Read the model definition and answer for the solid it produces. Units are mm, in the model's axes. Face numbers are marked on the shaded views. A direction names the side the tool comes from. Coordinates: 2 decimals unless noted, no trailing zeros. Loops run counter-clockwise (first coordinate to the right, second up) from the corner with the lowest first, then second, coordinate; pieces in that order, holes last. Notation, with made-up numbers: (69.5, -15.5) - (91.5, -15.5) arc R30 ccw to (91.5, 10.5) - close; hole circle Ø3 at (39, 44.5). An arc over 180 degrees is marked (long way). Use one line per item in the form item = value. Start each with the question number.
1) A cutting plane is placed at C-C (z = 6). State how many separate pieces and enclosed holes the cut face has, and give its area (3 significant figures).
2) A cutting plane is placed at A-A (y = 10). Give the vertices of the cut face in (x, z) (1 decimal).
3) The mould has two halves that part along X. Classify the marked faces 1, 2 and 3: released by +X, released by -X, zero draft, split by the parting line, or undercut.
4) Which of the six approach directions +Z, -Z, +X, -X, +Y, -Y give full straight-line access (tool end or side, diameter ignored) to the marked faces 4, 5 and 6?
5) A cutting plane is placed at B-B (y = 21.75). Give the vertices of the cut face in (x, z).
6) Consider line 1 (X direction, y = 16.5, z = 3); line 2 (X direction, y = 6.5, z = 6); line 3 (Z direction, x = 44, y = 22.75). Determine where each line is inside the solid, lowest interval first.
7) This flat-tipped pin is pushed along its axis until it touches: P1, Ø10, axis at x = -48, z = 4.5, coming from the -Y side (3 decimals). Where does it stop, or does it pass through?
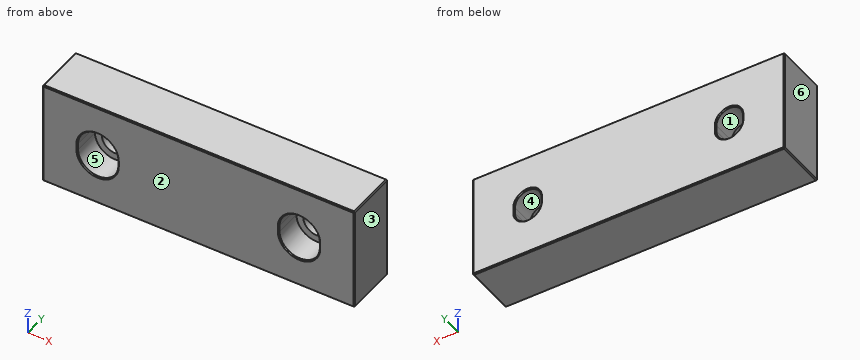
Autodesk Fusion 360 part; units mm, degrees
sketch "Sketch1" plane through (0, 0, 0) normal (0, 1, 0) x (1, 0, 0)
  line L0 (76.2, 25.4) -> (-76.2, 25.4)
  line L1 (-76.2, 25.4) -> (-76.2, -25.4)
  line L2 (-76.2, -25.4) -> (76.2, -25.4)
  line L3 (76.2, -25.4) -> (76.2, 25.4)
  line L4 (76.2, 25.4) -> (-76.2, -25.4) construction
  line L5 (-76.2, 25.4) -> (76.2, -25.4) construction
  line L6 (-55.6895, 1.524) -> (-55.6895, -1.524)
  arc A0 (-55.6895, -1.524) -> (-42.7355, -1.524) centre (-49.2125, -1.524) ccw
  line L7 (-42.7355, -1.524) -> (-42.7355, 1.524)
  arc A1 (-42.7355, 1.524) -> (-55.6895, 1.524) centre (-49.2125, 1.524) ccw
  line L8 (-49.2125, 1.524) -> (-49.2125, -1.524) construction
  line L9 (0, 0) -> (0, -13.116) construction
  line L10 (-59.055, 1.524) -> (-59.055, -1.524)
  arc A2 (-59.055, -1.524) -> (-39.37, -1.524) centre (-49.2125, -1.524) ccw
  line L11 (-39.37, -1.524) -> (-39.37, 1.524)
  arc A3 (-39.37, 1.524) -> (-59.055, 1.524) centre (-49.2125, 1.524) ccw
  line L12 (-49.2125, 1.524) -> (-49.2125, -1.524) construction
  arc A4 (39.37, -1.524) -> (59.055, -1.524) centre (49.2125, -1.524) ccw
  line L13 (39.37, -1.524) -> (39.37, 1.524)
  arc A5 (59.055, 1.524) -> (39.37, 1.524) centre (49.2125, 1.524) ccw
  line L14 (59.055, 1.524) -> (59.055, -1.524)
  line L15 (55.6895, 1.524) -> (55.6895, -1.524)
  arc A6 (42.7355, -1.524) -> (55.6895, -1.524) centre (49.2125, -1.524) ccw
  line L16 (42.7355, -1.524) -> (42.7355, 1.524)
  arc A7 (55.6895, 1.524) -> (42.7355, 1.524) centre (49.2125, 1.524) ccw
  point P0 (-49.2125, 0)
  point P1 (-49.2125, 0)
  dimension "d1" = 152.4
  dimension "d2" = 50.8
  dimension "d3" = 49.2125
  dimension "d4" = 19.685
  dimension "d5" = 12.954
  dimension "d6" = 23.876
  dimension "d7" = 23.876
extrude "Extrude1" add sketch "Sketch1" along normal blind 25.4 contours L0 L1 L2 L3 | L6 A0 L7 A1 | L10 A2 L11 A3 | A4 L13 A5 L14 | L15 A6 L16 A7
extrude "Extrude2" cut sketch "Sketch1" along normal through all contours L6 A0 L7 A1 | L15 A6 L16 A7
extrude "Extrude3" cut sketch "Sketch1" along normal up to surface (13.335 mm away) contours L10 A2 L11 A3 | A4 L13 A5 L14
chamfer "Chamfer1" distance 0.508 angle 45 28 edges at (0, 0, 25.4) (76.2, 0, 0) (0, 0, -25.4) (-76.2, 0, 0) (-76.2, 12.7, 25.4) (-76.2, 25.4, 0) (-76.2, 12.7, -25.4) (0, 25.4, -25.4) (0, 25.4, 25.4) (76.2, 25.4, 0) (76.2, 12.7, 25.4) (76.2, 12.7, -25.4) (49.2125, 0, -11.3665) (39.37, 0, 0) (49.2125, 0, 11.3665) (59.055, 0, 0) (-39.37, 0, 0) (-49.2125, 0, -11.3665) (-59.055, 0, 0) (-49.2125, 0, 11.3665) (-55.6895, 25.4, 0) (-49.2125, 25.4, -8.001) (-42.7355, 25.4, 0) (-49.2125, 25.4, 8.001) (42.7355, 25.4, 0) (49.2125, 25.4, -8.001) (55.6895, 25.4, 0) (49.2125, 25.4, 8.001)
equation "d7 = d6"
Found:
q1.separate_pieces = 3
q1.enclosed_holes = 0
q1.area = 3,180 mm^2
q2.outline = (-76.2, -24.9) - (-75.7, -25.4) - (75.7, -25.4) - (76.2, -24.9) - (76.2, 24.9) - (75.7, 25.4) - (-75.7, 25.4) - (-76.2, 24.9) - close; hole (-59.1, -1.5) arc R9.8 ccw to (-39.4, -1.5) - (-39.4, 1.5) arc R9.8 ccw to (-59.1, 1.5) - close; hole (39.4, -1.5) arc R9.8 ccw to (59.1, -1.5) - (59.1, 1.5) arc R9.8 ccw to (39.4, 1.5) - close
q3.face_1 = undercut
q3.face_2 = zero draft
q3.face_3 = released by +X
q4.face_4 = +Y, -Y
q4.face_5 = -Y
q4.face_6 = +Z, -Z, -X, +Y, -Y
q5.outline = (-76.2, -24.89) - (-75.69, -25.4) - (75.69, -25.4) - (76.2, -24.89) - (76.2, 24.89) - (75.69, 25.4) - (-75.69, 25.4) - (-76.2, 24.89) - close; hole (-55.69, -1.52) arc R6.48 ccw to (-42.74, -1.52) - (-42.74, 1.52) arc R6.48 ccw to (-55.69, 1.52) - close; hole (42.74, -1.52) arc R6.48 ccw to (55.69, -1.52) - (55.69, 1.52) arc R6.48 ccw to (42.74, 1.52) - close
q6.line_1 = -76.2 to -55.52, -42.91 to 42.91, 55.52 to 76.2
q6.line_2 = -76.2 to -57.98, -40.45 to 40.45, 57.98 to 76.2
q6.line_3 = -25.4 to -5.37, 5.37 to 25.4
q7.P1 = 13.335
